CAD build for the part. Positions are in the model's coordinates, mm. Round coordinates to 2 decimals unless told otherwise and drop trailing zeros. Write each loop counter-clockwise with the first axis right and the second up, starting at its lowest first coordinate (ties: lowest second). Pieces come first, ordered by that corner, then holes. Notation, with made-up numbers: (-15.5, 83.25) - (3.5, 83.25) arc R21 cw to (3.5, 121.25) - close; hole circle Ø1 at (74.5, 6). An arc over 180 degrees is marked (long way). Use one line per item in the form item = value. Start each with the question number.
Item 1: Pin check, flat tips, straight feed: pin 1 (9 mm diameter, centred on x = -19.05, y = 3.175, fed in from -Z) (3 decimals); pin 2 (4 mm diameter, centred on x = 19.05, y = 3.175, fed in from -Z). Stop position of each tip, or through.
Item 2: Band-saw the part on A-A, the plane x = -19.05. List the corners of the cut face in (y, z) (3 decimals), and give its area (3 significant figures).
Item 3: Drill centre lines: L1, parallel to Y at x = -19.05, z = -1.35 (3 decimals); L2, parallel to X at y = -1, z = 0.5 (3 decimals); L3, parallel to X at y = 5, z = -0.4 (3 decimals). Where is each one in solid material? Low to high.
Item 4: Pull direction Y, two halves, no side cores. Call faces 1 (the flat face through (0, 22.225, 0)), 2 (the flat face through (0, 0, -2.375)), 3 (the flat face through (0, -22.225, 0)), 4 (the conical face through (22.589, 3.64, -0.926)): +Y half, -Y half, draft (parallel to the pull), parting line (faces both ways), or undercut.
Item 5: Band-saw the part on B-B, the plane z = 0.3. List the corners of the cut face in (x, y) (3 decimals), and give its area (3 significant figures).
from build123d import *

# Parameters (mm, degrees)
SKETCH1_W           = 69.85
SKETCH1_H           = 44.45
BOSS_EXTRUDE1_DEPTH = 2.375


with BuildPart() as part:
    # Sketch1 → Boss-Extrude1 (new, symmetric)
    with BuildSketch(Plane.XY):
        Rectangle(SKETCH1_W, SKETCH1_H)
    extrude(amount=BOSS_EXTRUDE1_DEPTH, both=True)

    # Sketch4 → CSK for 1/4 Flat Head Machine Screw1 (revolve, cut)
    with BuildSketch(Plane(origin=(-19.05, 3.175, 2.375), x_dir=(0, -1, 0), z_dir=(1, 0, 0))):
        Polygon((0, 0), (0, 4.75), (3.3782, 4.75), (3.3782, 3.520932584), (6.4389, 0), align=None)
    csk_for_1_4_flat_head_machine_screw1 = revolve(axis=Axis((-19.05, 3.175, 8.725), (0, 0, -1)), mode=Mode.SUBTRACT)

    # Mirror1: CSK for 1/4 Flat Head Machine Screw1 across plane
    add(csk_for_1_4_flat_head_machine_screw1.mirror(Plane(origin=(0, 0, 0), x_dir=(0, 0, 1), z_dir=(1, 0, 0))), mode=Mode.SUBTRACT)


solid = part.part
Determined:
q1.pin_1 = -2.375
q1.pin_2 = through
q2.outline = (-22.225, -2.375) - (-0.203, -2.375) - (-0.203, -1.146) - (-3.264, 2.375) - (-22.225, 2.375) - close; (6.553, -2.375) - (22.225, -2.375) - (22.225, 2.375) - (9.614, 2.375) - (6.553, -1.146) - close
q2.area = 168 mm²
q3.L1 = -22.225 to -0.203, 6.553 to 22.225
q3.L2 = -34.925 to -21.437, -16.663 to 16.663, 21.437 to 34.925
q3.L3 = -34.925 to -22.639, -15.461 to 15.461, 22.639 to 34.925
q4.face_1 = +Y half
q4.face_2 = draft
q4.face_3 = -Y half
q4.face_4 = undercut
q5.outline = (-34.925, -22.225) - (34.925, -22.225) - (34.925, 22.225) - (-34.925, 22.225) - close; hole circle Ø9.27 at (-19.05, 3.175); hole circle Ø9.27 at (19.05, 3.175)
q5.area = 2,970 mm²
